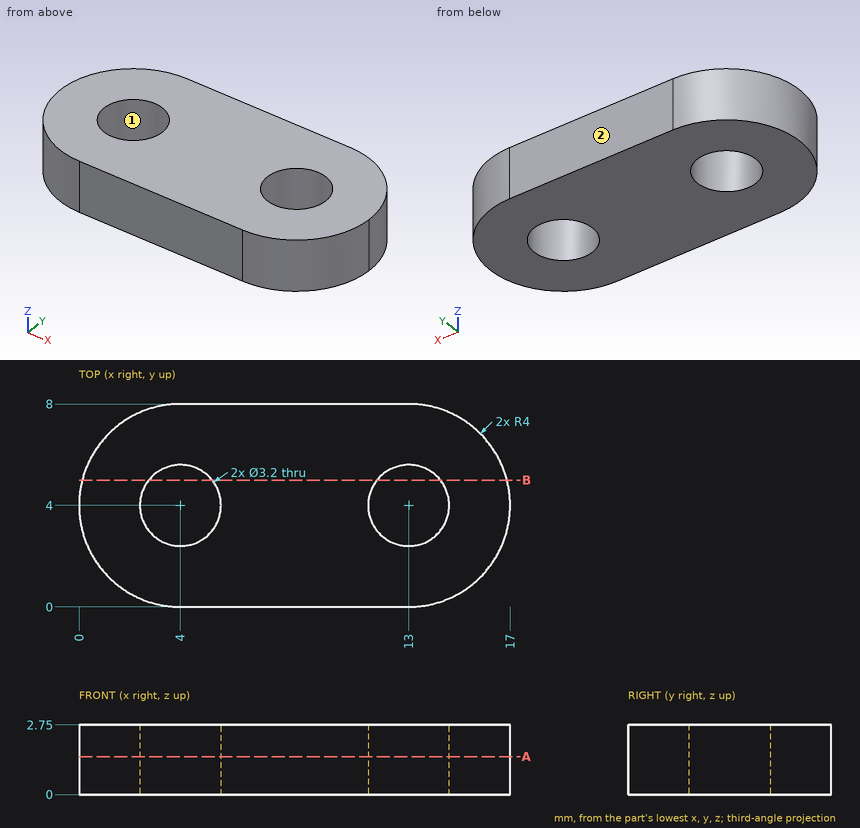
Geometry: see drawing. Coordinates: mm, zero at the bounding-box minimum. Coordinates: 2 decimals unless noted, no trailing zeros. Order: outer loops, then holes, each group sorted by start corner. A loop starts at its lowest first (then second) coordinate and runs counter-clockwise, first axis right, second up. Notation, with made-up numbers: (43.5, -20.75) - (48.5, -20.75) arc R16 cw to (48.5, 2.25) - close; hole circle Ø5 at (-19.5, -4). An arc over 180 degrees is marked (long way). Write each question's results on one line, items separated by ' | '.
1) Section B-B, the plane y = 5. Return loops of the section in (x, z), plus the area to 3 significant figures.
Results list:
outline: (0.13, 0) - (2.75, 0) - (2.75, 2.75) - (0.13, 2.75) - close; (5.25, 0) - (11.75, 0) - (11.75, 2.75) - (5.25, 2.75) - close; (14.25, 0) - (16.87, 0) - (16.87, 2.75) - (14.25, 2.75) - close | area: 32.3 mm^2
2) Line query: line 1 (X direction, y = 3.5, z = 0.7); line 2 (Y direction, x = 12.5, z = 0.2); line 3 (Y direction, x = 3.25, z = 2.45). Output: solid intervals per line, ascending. Write a range as from..to.
Results list:
line 1: 0.03..2.48, 5.52..11.48, 14.52..16.97 | line 2: 0..2.48, 5.52..8 | line 3: 0.07..2.59, 5.41..7.93
3) Pull-direction query (X, two-part tool) for the marked faces 1 and 2; classes: pulls with the +X half, pulls with the -X half, needs draft (parallel to the pull), parting line crosses it, or undercut.
Results list:
face 1: undercut | face 2: needs draft
4) Pin query (flat end, axial travel): pin 1 (1 mm diameter, centred on y = 2.5, z = 2, fed in from +X). Return the tip coordinate at first contact, or that it passes through.
Results list:
pin 1: x = 16.87
5) Section A-A, the plane z = 1.5. Return loops of the section in (x, y).
Results list:
outline: (4, 0) - (13, 0) arc R4 ccw to (13, 8) - (4, 8) arc R4 ccw to start; hole circle Ø3.2 at (4, 4); hole circle Ø3.2 at (13, 4)
